Model file for the job. Use its own axes, mm. A direction names the side the tool comes from. Give positions to 0.01 mm unless a question says otherwise; leave off trailing zeros. Loops run counter-clockwise (first coordinate to the right, second up) from the corner with the lowest first, then second, coordinate; pieces in that order, holes last. Notation, with made-up numbers: (-14.5, -14) -> (1.5, -14) arc R8 ccw to (1.5, -5) -> close; hole circle Ø8 at (62, 48.5). An arc over 180 degrees is marked (long way). Use CSV: the item, a comma, the result in double quotes. Start each with the question number.
(1) Pull direction Z, two halves, no side cores. Call faces 3 (the flat face through (0, 8, -14.25)), 4 (the flat face through (-10.75, 7, 0)), 5 (the cylindrical face through (-0.02, -0.99, -12.75)): pulls with the +Z half, pulls with the -Z half, needs draft (parallel to the pull), parting line crosses it, or undercut.
(2) 3-axis set-ups, long thin cutter, end or side, ignore diameter. For faces 1 (the flat face through (0, -2, 12)), 2 (the cylindrical face through (-0.02, -0.99, 11.75)): which of +Z, -Z, +X, -X, +Y, -Y reach the whole face in a straight line?
(3) Cut at B-B on x = 0. Write the cut outline in (y, z).
(4) Cut at C-C on z = 12.25. Write the cut outline in (x, y).
(5) Cut at A-A on z = 2.5. Write the cut outline in (x, y).
(6) Cut at D-D on x = -7.5. Write the cut outline in (y, z).
(7) Drill centre lines: probe 1 along Y at (x, z) = (-2, -5); probe 2 along Y at (x, z) = (-9, -8.25); probe 3 along X at (y, z) = (14.5, -0.75). Where is each one in solid material? Low to high.
from build123d import *

# Parameters (mm, degrees)
EXTRUDE_2_DEPTH = 14.25
SKETCH_2_R      = 0.5
EXTRUDE_3_DEPTH = 2


with BuildPart() as part:
    # Эскиз1 → Бобышка-Вытянуть2 (new, symmetric)
    with BuildSketch(Plane.XY):
        Polygon((-10.75, 0), (10.75, 0), (10.75, 14), (8.75, 16), (-8.75, 16), (-10.75, 14), align=None)
    extrude(amount=EXTRUDE_2_DEPTH, both=True)

    # Эскиз2 → Бобышка-Вытянуть3 (add)
    with BuildSketch(Plane.XZ):
        with Locations(Location((0, 12.25, 0), (0, 0, 90))):
            Circle(SKETCH_2_R)
        with Locations(Location((0, -12.25, 0), (0, 0, 90))):
            Circle(SKETCH_2_R)
    extrude(amount=EXTRUDE_3_DEPTH)


solid = part.part
Check result:
1,face 3,"pulls with the -Z half"
1,face 4,"needs draft"
1,face 5,"undercut"
2,face 1,"+Z, -Z, +X, -X, -Y"
2,face 2,"-Y"
3,outline,"(-2, -12.75) -> (0, -12.75) -> (0, -14.25) -> (16, -14.25) -> (16, 14.25) -> (0, 14.25) -> (0, 12.75) -> (-2, 12.75) -> (-2, 11.75) -> (0, 11.75) -> (0, -11.75) -> (-2, -11.75) -> close"
4,outline,"(-10.75, 0) -> (-0.5, 0) -> (-0.5, -2) -> (0.5, -2) -> (0.5, 0) -> (10.75, 0) -> (10.75, 14) -> (8.75, 16) -> (-8.75, 16) -> (-10.75, 14) -> close"
5,outline,"(-10.75, 0) -> (10.75, 0) -> (10.75, 14) -> (8.75, 16) -> (-8.75, 16) -> (-10.75, 14) -> close"
6,outline,"(0, -14.25) -> (16, -14.25) -> (16, 14.25) -> (0, 14.25) -> close"
7,probe 1,"0 to 16"
7,probe 2,"0 to 15.75"
7,probe 3,"-10.25 to 10.25"
